Verification items for the finished model (mm, model axes). A direction names the side the tool comes from. Round coordinates to 2 decimals unless told otherwise and drop trailing zeros. Loops run counter-clockwise (first coordinate to the right, second up) from the corner with the lowest first, then second, coordinate; pieces in that order, holes last. Notation, with made-up numbers: (-13.75, -19) - (45.25, -19) arc R8 ccw to (45.25, -10) - close; hole circle Ø10 at (29.25, 83.25). An arc over 180 degrees is marked (long way). Use a Markdown table: item, result. Add a question column.
```python
from build123d import *

# Parameters (mm, degrees)
F1_DEPTH = 20
F2_R     = 4
F3_DEPTH = 65.2
F4_R     = 9.99999
F5_R     = 2
F7_D     = 2.5
F8_D     = 6


# Not quite as in the source:
# - a fillet or chamfer is up to 0.001 mm smaller than in the source, because OpenCascade refuses the exact size


with BuildPart() as f1:
    # F0 (on Front) → F1 (new body)
    with BuildSketch(Plane.XZ):
        Polygon((-25.5, 37), (-27.5, 37), (-27.5, 0), (27.5, 0), (27.5, 37), (25.5, 37), (25.5, 2), (-25.5, 2), align=None)
    extrude(amount=F1_DEPTH)

    # F2 (on face) → F3 (cut)
    with BuildSketch(Plane(origin=(-27.5, 0, 0), x_dir=(0, -1, 0), z_dir=(-1, 0, 0))):
        with Locations((10, 27)):
            Circle(F2_R)
    extrude(amount=-F3_DEPTH, mode=Mode.SUBTRACT)

    # F4 (radius 10 in the source; OpenCascade refuses exactly that, so slightly less here)
    f4_edges = [f1.edges().sort_by_distance(p)[0] for p in [
        (-26.5, 0, 37),
        (-26.5, -20, 37),
        (26.5, 0, 37),
        (26.5, -20, 37),
    ]]
    fillet(f4_edges, radius=F4_R)

    # F5
    f5_edges = [f1.edges().sort_by_distance(p)[0] for p in [
        (-27.5, -10, 0),
        (27.5, -10, 0),
    ]]
    fillet(f5_edges, radius=F5_R)

    # F7 (through all)
    with Locations(Plane(origin=(0, 0, 0), x_dir=(1, 0, 0), z_dir=(0, 0, -1))):
        with Locations((-15, 15), (-5, 15), (5, 15), (15, 15), (-15, 5), (-5, 5), (5, 5), (15, 5)):
            Hole(F7_D / 2)

    # F8 (through all)
    with Locations(Plane(origin=(0, 0, 0), x_dir=(1, 0, 0), z_dir=(0, 0, -1))):
        with Locations((0, 10)):
            Hole(F8_D / 2)


solid = f1.part
```
Q1. Section check D-D on y = -9.25. Record the cut outline in (x, z).
Q2. Go/stop test with flat-tipped pins: pin 1 Ø4 at (x, y) = (15, -15) entering from +Z; pin 2 Ø5 at (y, z) = (-10, 27) entering from -X. Record where each tip stops, or that it passes through.
Q3. Thickness scan on line 1 along Y through (x, z) = (-5, 1); line 2 along X through (y, z) = (-18.5, 15.5); line 3 along X through (y, z) = (-15, 0.85). Record the ranges inside material, lowest first.
Q4. Set-up check for faces 4 (the face through (3, -10, 1)), 5 (the face through (25.5, -10, 20)): record each of +Z, -Z, +X, -X, +Y, -Y from which the full face is reachable in a straight line by a thin tool's end or side.
Q5. Release check for a two-part mould opening along Y. For faces 1 (the face through (-26.51, -16.99, 34.15)), 2 (the face through (-27.5, -10, 20)), 3 (the face through (-14.079, -15.845, 1.014)) record: +Y half, -Y half, draft (parallel to the pull), parting line (faces both ways), or undercut.
Q6. Section check C-C on z = 21. Record the cut outline in (x, y), plus the area to 3 significant figures.
Q7. Section check B-B on y = -5. Record the cut outline in (x, z).
Q8. Section check A-A on x = 5. Record the cut outline in (y, z).
Determined:
| question | item | result |
|---|---|---|
| 1 | outline | (-27.5, 2) arc R2 ccw to (-25.5, 0) - (-2.9, 0) - (-2.9, 2) - (-25.5, 2) - (-25.5, 23.07) - (-27.5, 23.07) - close; (-27.5, 30.93) - (-25.5, 30.93) - (-25.5, 36.97) - (-27.5, 36.97) - close; (2.9, 0) - (25.5, 0) arc R2 ccw to (27.5, 2) - (27.5, 23.07) - (25.5, 23.07) - (25.5, 2) - (2.9, 2) - close; (25.5, 30.93) - (27.5, 30.93) - (27.5, 36.97) - (25.5, 36.97) - close |
| 2 | pin 1 | stops at z = 2 |
| 2 | pin 2 | passes through |
| 3 | line 1 | y = -20 to -16.25, -13.75 to -6.25, -3.75 to 0 |
| 3 | line 2 | x = -27.5 to -25.5, 25.5 to 27.5 |
| 3 | line 3 | x = -27.14 to -16.25, -13.75 to -6.25, -3.75 to 3.75, 6.25 to 13.75, 16.25 to 27.14 |
| 4 | face 4 | +Z, -Z |
| 4 | face 5 | +Z, +Y, -Y |
| 5 | face 1 | -Y half |
| 5 | face 2 | draft |
| 5 | face 3 | undercut |
| 6 | outline | (-27.5, -20) - (-25.5, -20) - (-25.5, 0) - (-27.5, 0) - close; (25.5, -20) - (27.5, -20) - (27.5, 0) - (25.5, 0) - close |
| 6 | area | 80.0 mm² |
| 7 | outline | (-27.5, 2) arc R2 ccw to (-25.5, 0) - (-16.25, 0) - (-16.25, 2) - (-25.5, 2) - (-25.5, 35.66) - (-27.5, 35.66) - close; (-13.75, 0) - (-6.25, 0) - (-6.25, 2) - (-13.75, 2) - close; (-3.75, 0) - (3.75, 0) - (3.75, 2) - (-3.75, 2) - close; (6.25, 0) - (13.75, 0) - (13.75, 2) - (6.25, 2) - close; (16.25, 0) - (25.5, 0) arc R2 ccw to (27.5, 2) - (27.5, 35.66) - (25.5, 35.66) - (25.5, 2) - (16.25, 2) - close |
| 8 | outline | (-20, 0) - (-16.25, 0) - (-16.25, 2) - (-20, 2) - close; (-13.75, 0) - (-6.25, 0) - (-6.25, 2) - (-13.75, 2) - close; (-3.75, 0) - (0, 0) - (0, 2) - (-3.75, 2) - close |
